Geometry: final body of the model. Coordinates: model frame, mm. Give positions to 0.01 mm unless a question says otherwise; leave off trailing zeros. Write each loop counter-clockwise with the first axis right and the second up, starting at its lowest first coordinate (ties: lowest second). Pieces come first, ordered by that corner, then holes. Notation, with made-up numbers: M 16.5,20 L 63.5,20 A22 cw 63.5,57 Z; hole C 85,38.5 d11. An arc over 180 degrees is marked long. Use a Markdown table: item, result. Add a question column.
1) Line query: line 1 (Z direction, x = 0, y = -16); line 2 (X direction, y = -5.5, z = 19.5); line 3 (Z direction, x = -11, y = -2). Output: solid intervals per line, ascending.
2) Section D-D on x = 22. Return the cut outline in (y, z).
3) Section B-B on y = -5.5. Return the cut outline in (x, z), then the cut area to 3 significant figures.
4) Section C-C on x = -9.5. Return the cut outline in (y, z).
5) Pin query (flat end, axial travel): pin 1 (12 mm diameter, centred on x = 8, y = -20.5, fed in from +Z); pin 2 (12 mm diameter, centred on x = 12, z = 26.5, fed in from +Y). Return the tip coordinate at first contact, or that it passes through.
6) Draft query along X for faces 1 (the cylindrical face through (-9.64, -15.65, 12.08)), 2 (the flat face through (25.372, -16, -13)), 3 (the flat face through (-25.372, -16, -12)). Return one class per face: +X half, -X half, draft (parallel to the pull), parting line (faces both ways), or undercut.
7) Section A-A on x = 0. Return the cut outline in (y, z).
```python
from build123d import *

# Parameters (mm, degrees)
F0_R     = 12.145275
F1_DEPTH = 31.75


with BuildPart() as f1:
    # F0 (on Front) → F1 (new body)
    with BuildSketch(Plane.XZ):
        with BuildLine():
            ThreePointArc((25.372297, 19.465521), (-1e-06, 44.837818), (-25.372298, 19.465521))
            Line((-25.372298, 19.465521), (-25.372298, -45.240555))
            Line((-25.372298, -45.240555), (25.372297, -45.240555))
            Line((25.372297, -45.240555), (25.372297, 19.465521))
        make_face()
        with Locations((-1e-06, 19.465521)):
            Circle(F0_R, mode=Mode.SUBTRACT)
    extrude(amount=F1_DEPTH)


solid = f1.part
```
Found:
| question | item | result |
|---|---|---|
| 1 | line 1 | -45.24 to 7.32, 31.61 to 44.84 |
| 1 | line 2 | -25.37 to -12.15, 12.15 to 25.37 |
| 1 | line 3 | -45.24 to 14.32, 24.61 to 42.33 |
| 2 | outline | M -31.75,-45.24 L 0,-45.24 L 0,32.1 L -31.75,32.1 Z |
| 3 | outline | M -25.37,-45.24 L 25.37,-45.24 L 25.37,19.47 A25.37 ccw -25.37,19.47 Z; hole C 0,19.47 d24.29 |
| 3 | area | 3,830 mm² |
| 4 | outline | M -31.75,-45.24 L 0,-45.24 L 0,11.9 L -31.75,11.9 Z; M -31.75,27.03 L 0,27.03 L 0,42.99 L -31.75,42.99 Z |
| 5 | pin 1 | z = 44.76 |
| 5 | pin 2 | y = 0 |
| 6 | face 1 | undercut |
| 6 | face 2 | +X half |
| 6 | face 3 | -X half |
| 7 | outline | M -31.75,-45.24 L 0,-45.24 L 0,7.32 L -31.75,7.32 Z; M -31.75,31.61 L 0,31.61 L 0,44.84 L -31.75,44.84 Z |
